Job drawing, mm, ordinate dimensions from the low corner. One solid piece. A direction names the side the tool comes from. Give positions to 0.01 mm unless a question says otherwise; leave off trailing zeros. Order: outer loops, then holes, each group sorted by start corner. A loop starts at its lowest first (then second) coordinate and runs counter-clockwise, first axis right, second up. Notation, with made-up numbers: M 50,-10.75 L 103,-10.75 A28 ccw 103,10.25 Z; hole C 49.25,82.25 d3. An arc over 180 degrees is marked long. One line per question, with ' | ' between items.
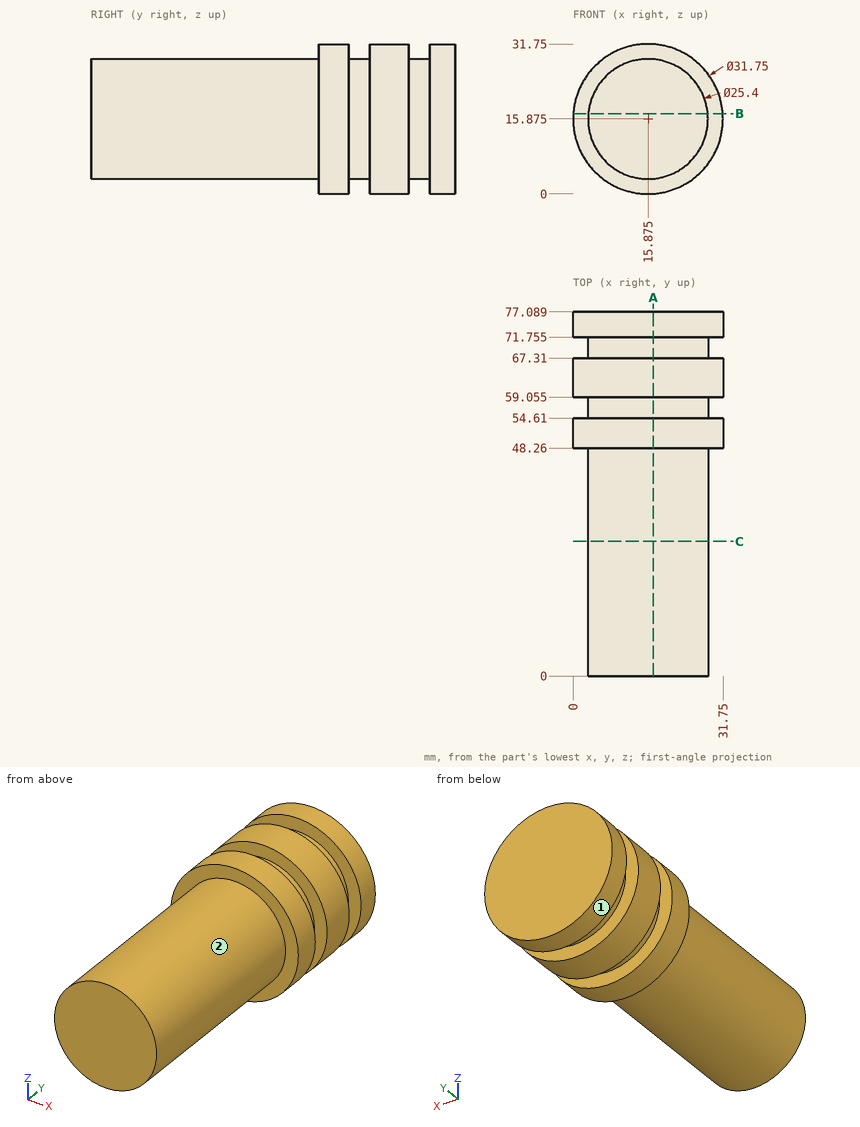
1. Slice it at C-C on y = 28.5. Give the cut face in (x, z) (3 decimals).
Worked out:
outline: C 15.875,15.875 d25.4
2. Slice it at A-A on x = 17. Give the cut face in (y, z) (3 decimals).
Worked out:
outline: M 0,3.225 L 48.26,3.225 L 48.26,0.04 L 54.61,0.04 L 54.61,3.225 L 59.055,3.225 L 59.055,0.04 L 67.31,0.04 L 67.31,3.225 L 71.755,3.225 L 71.755,0.04 L 77.089,0.04 L 77.089,31.71 L 71.755,31.71 L 71.755,28.525 L 67.31,28.525 L 67.31,31.71 L 59.055,31.71 L 59.055,28.525 L 54.61,28.525 L 54.61,31.71 L 48.26,31.71 L 48.26,28.525 L 0,28.525 Z
3. Drop flat-ended pins along their axis: pin 1 (2 mm diameter, centred on x = 27.5, y = 67.5, fed in from -Z); pin 2 (1.5 mm diameter, centred on x = 9, y = 9, fed in from +Z); pin 3 (9.5 mm diameter, centred on x = 12, z = 19.5, fed in from -Y); pin 4 (6 mm diameter, centred on x = 9.5, y = 68, fed in from -Z). Give the stop position or say it passes through.
Worked out:
pin 1: stops at z = 4.1 | pin 2: stops at z = 27 | pin 3: stops at y = 0 | pin 4: stops at z = 0.38
4. Slice it at B-B on z = 17. Give the cut face in (x, y) (3 decimals).
Worked out:
outline: M 0.04,48.26 L 3.225,48.26 L 3.225,0 L 28.525,0 L 28.525,48.26 L 31.71,48.26 L 31.71,54.61 L 28.525,54.61 L 28.525,59.055 L 31.71,59.055 L 31.71,67.31 L 28.525,67.31 L 28.525,71.755 L 31.71,71.755 L 31.71,77.089 L 0.04,77.089 L 0.04,71.755 L 3.225,71.755 L 3.225,67.31 L 0.04,67.31 L 0.04,59.055 L 3.225,59.055 L 3.225,54.61 L 0.04,54.61 Z
5. Probe L1, parallel to Y at x = 11, z = 3 (3 decimals); L2, parallel to X at y = 47.5, z = 16.5; L3, parallel to Z at x = 16.5, y = 60. List the from-to ranges inside material, lowest first. Write a range as from..to.
Worked out:
L1: y = 48.26..54.61, 59.055..67.31, 71.755..77.089 | L2: x = 3.19..28.56 | L3: z = 0.01..31.74
6. Tool access for the marked faces 1 and 2: list every direction of +Z, -Z, +X, -X, +Y, -Y with a clear straight run to the whole face (end or side of a thin tool).
Worked out:
face 1: +Y, -Y | face 2: -Y
